Check sheet for the modelled part. Datum: model origin and axes. Units: mm. A direction names the side the tool comes from. Round coordinates to 2 decimals unless told otherwise and drop trailing zeros. Order: outer loops, then holes, each group sorted by start corner. A loop starts at its lowest first (then second) coordinate and runs counter-clockwise, first axis right, second up.
Autodesk Inventor part; units mm, degrees
ref_plane "YZ Plane" through (0, 0, 0) normal (1, 0, 0) x (0, 1, 0)
ref_plane "XZ Plane" through (0, 0, 0) normal (0, 1, 0) x (-1, 0, 0)
ref_plane "XY Plane" through (0, 0, 0) normal (0, 0, 1) x (1, 0, 0)
sketch "Boceto1" plane through (0, 0, 0) normal (0, 1, 0) x (-1, 0, 0)
  line L0 (0, 0) -> (100, 0)
  line L1 (100, 0) -> (100, -130)
  line L2 (100, -130) -> (0, -130)
  line L3 (0, -130) -> (0, 0)
  dimension "d0" = 100
  dimension "d1" = 130
extrude "Extrusión1" add sketch "Boceto1" along normal blind 28
sketch "Boceto2" plane through (0, 28, 0) normal (0, 1, 0) x (1, 0, 0)
  line L0 (-70, 13.56) -> (-30, 13.56)
  line L1 (-30, 13.56) -> (-30, 14.36)
  line L2 (-30, 14.36) -> (-70, 14.36)
  line L3 (-70, 14.36) -> (-70, 13.56)
  line L4 (-100, 0) -> (0, 0)
  line L5 (0, 0) -> (0, 130)
  line L6 (-70, 16.36) -> (-30, 16.36)
  line L7 (-30, 16.36) -> (-30, 17.26)
  line L8 (-30, 17.26) -> (-70, 17.26)
  line L9 (-70, 17.26) -> (-70, 16.36)
  line L10 (-70, 19.26) -> (-30, 19.26)
  line L11 (-30, 19.26) -> (-30, 20.16)
  line L12 (-30, 20.16) -> (-70, 20.16)
  line L13 (-70, 20.16) -> (-70, 19.26)
  line L14 (-85, 85) -> (-15, 85)
  line L15 (-15, 85) -> (-15, 35)
  line L16 (-15, 35) -> (-85, 35)
  line L17 (-85, 35) -> (-85, 85)
  line L18 (-100, 130) -> (-100, 0)
  line L19 (0, 130) -> (-100, 130)
  circle A0 centre (-50, 107.5) radius 4.5
  dimension "d4" = 40
  dimension "d5" = 0.8
  dimension "d6" = 13.56
  dimension "d7" = 30
  dimension "d8" = 40
  dimension "d9" = 0.9
  dimension "d10" = 2
  dimension "d11" = 0
  dimension "d12" = 40
  dimension "d13" = 0.9
  dimension "d14" = 0
  dimension "d15" = 2
  dimension "d16" = 70
  dimension "d17" = 50
  dimension "d18" = 15
  dimension "d19" = 45
  dimension "d20" = 9
  dimension "d21" = 50
  dimension "d22" = 22.5
extrude "Extrusión2" cut sketch "Boceto2" against normal blind 28 contours L3 L2 L1 L0 | L9 L8 L7 L6 | L13 L12 L11 L10 | L14 L15 L16 L17 | A0
equation "\"Radio_pliegue\" = Grosor"
equation "\"Anchura_desahogo_plegado\" = Grosor"
equation "\"Profundidad_desahogo_plegado\" = 0.5 * Grosor"
equation "\"Tamaño_destalonado\" = 4 * Grosor"
equation "\"Remanente_mínimo\" = 2 * Grosor"
equation "\"Radiodetransición\" = Radio_pliegue"
equation "\"Tamaño_de_radio_de_Jacobi\" = Radio_pliegue"
equation "\"TamañoSeparación\" = Grosor"
properties part number "carcasaV1"
Item 1: Access from +Z, -Z, +X, -X, +Y, -Y to the whole of each face (thin tool, end or side, straight path). Record for faces 1 (the flat face through (-49, 14, 0)), 2 (the flat face through (-50, 14, -16.36)).
Answer:
face 1: +Z, +X, -X, +Y, -Y
face 2: +Y, -Y
Item 2: Sectioned sample at C-C (y = 13.75). Record the cut outline in (x, z), and give its area (3 significant figures).
Answer:
outline: (-100, -130) - (0, -130) - (0, 0) - (-100, 0) - close; hole (-85, -85) - (-15, -85) - (-15, -35) - (-85, -35) - close; hole (-70, -20.16) - (-30, -20.16) - (-30, -19.26) - (-70, -19.26) - close; hole (-70, -17.26) - (-30, -17.26) - (-30, -16.36) - (-70, -16.36) - close; hole (-70, -14.36) - (-30, -14.36) - (-30, -13.56) - (-70, -13.56) - close; hole circle Ø9 at (-50, -107.5)
area: 9,330 mm2
Item 3: Scan lines: line 1 along Z through (x, y) = (-50, 14); line 2 along X through (y, z) = (20.25, -107.5); line 3 along X through (y, z) = (7.25, -42.5). Record each from-to range of solid material in increasing order.
Answer:
line 1: z = -130 to -112, -103 to -85, -35 to -20.16, -19.26 to -17.26, -16.36 to -14.36, -13.56 to 0
line 2: x = -100 to -54.5, -45.5 to 0
line 3: x = -100 to -85, -15 to 0
Item 4: Sectioned sample at A-A (x = -50). Record the cut outline in (y, z), and give its area (3 significant figures).
Answer:
outline: (0, -130) - (28, -130) - (28, -112) - (0, -112) - close; (0, -103) - (28, -103) - (28, -85) - (0, -85) - close; (0, -35) - (28, -35) - (28, -20.16) - (0, -20.16) - close; (0, -19.26) - (28, -19.26) - (28, -17.26) - (0, -17.26) - close; (0, -16.36) - (28, -16.36) - (28, -14.36) - (0, -14.36) - close; (0, -13.56) - (28, -13.56) - (28, 0) - (0, 0) - close
area: 1,920 mm2
Item 5: Sectioned sample at D-D (x = -74.5). Record the cut outline in (y, z).
Answer:
outline: (0, -130) - (28, -130) - (28, -85) - (0, -85) - close; (0, -35) - (28, -35) - (28, 0) - (0, 0) - close
Item 6: Sectioned sample at B-B (z = -52.5). Record the cut outline in (x, y).
Answer:
outline: (-100, 0) - (-85, 0) - (-85, 28) - (-100, 28) - close; (-15, 0) - (0, 0) - (0, 28) - (-15, 28) - close
Item 7: Release check for a two-part mould opening along X. For faces 3 (the flat face through (-100, 14, -64)), 4 (the flat face through (-15, 14, -60)), 5 (the flat face through (-49, 0, -93)) record: released by +X, released by -X, zero draft, split by the parting line, or undercut.
Answer:
face 3: released by -X
face 4: undercut
face 5: zero draft
